Here's how the part is built. I have some questions about the finished solid (model axes, mm). Face numbers are marked on the shaded views. A direction names the side the tool comes from. Give positions to 0.01 mm unless a question says otherwise; leave off trailing zeros. Loops run counter-clockwise (first coordinate to the right, second up) from the corner with the lowest first, then second, coordinate; pieces in that order, holes last. Notation, with made-up numbers: M 73.5,55 L 77.5,55 A24 ccw 77.5,69 Z; hole C 73.5,31 d5. An arc over 180 degrees is marked long. Write item = value, one per line. Start each with the question number.
Autodesk Inventor part; units mm, degrees
ref_plane "YZ Plane" through (0, 0, 0) normal (1, 0, 0) x (0, 1, 0)
ref_plane "XZ Plane" through (0, 0, 0) normal (0, 1, 0) x (-1, 0, 0)
ref_plane "XY Plane" through (0, 0, 0) normal (0, 0, 1) x (1, 0, 0)
sketch "Sketch1" plane through (0, 0, 0) normal (0, 0, 1) x (1, 0, 0)
  line L0 (0, 0) -> (0, 25.4713) construction
  line L1 (-206.1253, 8.0706) -> (-206.1253, -17.3294)
  line L2 (-206.1253, -17.3294) -> (-203.2, -23.287)
  line L3 (-203.2, -23.287) -> (-203.2, -17.3294)
  line L4 (-203.2, -17.3294) -> (-196.85, -17.3294)
  line L5 (-196.85, -17.3294) -> (-196.85, -18.6213)
  line L6 (-206.1253, 8.0706) -> (-202.8327, 15.2137)
  line L7 (-202.8327, 15.2137) -> (-202.8327, 8.0706)
  line L8 (-202.8327, 8.0706) -> (-196.8015, 8.0706)
  line L9 (-196.8015, 8.0706) -> (-196.8015, 9.3626)
  line L10 (-196.8015, 9.3626) -> (-177.369, 9.3626)
  line L11 (-196.85, -18.6213) -> (-177.4174, -18.6213)
  line L12 (-159.6027, 47.4626) -> (-196.85, 47.4626)
  line L13 (-196.85, 47.4626) -> (-196.85, 71.7094)
  line L14 (-196.85, 71.7094) -> (-148.2962, 71.7094)
  line L15 (-159.6511, -56.7213) -> (-195.9938, -56.7213)
  line L16 (-195.9938, -56.7213) -> (-195.9938, -78.0553)
  line L17 (-195.9938, -78.0553) -> (-149.7029, -78.0553)
  line L18 (-177.369, 9.3626) -> (-159.6027, 47.4626)
  line L19 (-148.2962, 71.7094) -> (-143.6137, 81.751)
  line L20 (-177.4174, -18.6213) -> (-159.6511, -56.7213)
  line L21 (-149.7029, -78.0553) -> (-143.013, -92.4018)
  line L22 (-143.6137, 81.751) -> (-114.6581, 143.8464)
  line L23 (-143.013, -92.4018) -> (-109.7002, -163.8414)
  line L24 (-114.6581, 143.8464) -> (-88.6327, 143.8464)
  line L25 (-88.6327, 143.8464) -> (-88.6327, -163.8414)
  line L26 (-88.6327, -163.8414) -> (-109.7002, -163.8414)
  dimension "d0" = 6.35
  dimension "d3" = 203.2
  dimension "d11" = 38.1
  dimension "d12" = 38.1
  dimension "d13" = 0
  dimension "d14" = 25.4
  dimension "d15" = 0
  dimension "d16" = 115
  dimension "d17" = 115
revolve "Revolution1" add sketch "Sketch1" angle 360 about axis through (0, 0, 0) along (0, 1, 0)
properties part number "Section Adaptor WIP"
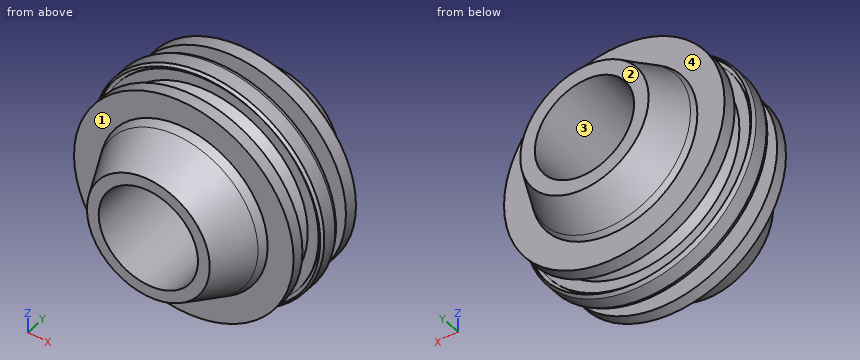
Q1. On a 3-axis mill with a long thin cutter (end or side, diameter ignored), from which of +Z, -Z, +X, -X, +Y, -Y can I reach the whole of each face in a straight line? I mean the marked faces 1 and 2. Say none if no direction works.
Q2. If we section it at A-A, the plane y = 55: List the corners of the cut face in (x, z) for me, then the cut area to 3 significant figures.
Q3. If we section it at B-B, the plane x = 164: State how many separate pieces and enclosed holes the cut face has, then the cut area to 3 significant figures.
Q4. If I drill on line 1 along Y through (x, z) = (140.5, -121); line 2 along Y through (x, z) = (50.5, 153); line 3 along Z through (x, y) = (0, 10.75), over which ranges is the centre line in solid material (lowest first)?
Q5. We'd pull the mould along Z, two halves only. Please class the marked faces 3 and 4: pulls with the +Z half, pulls with the -Z half, needs draft (parallel to the pull), parting line crosses it, or undercut.
Q6. If we section it at C-C, the plane y = 1: List the corners of the cut face in (x, z) for me.
Q7. Will these pins go through, and if not, where does the flat tip stop? pin 1 (12 mm diameter, centred on x = -49, y = 82, fed in from -Z); pin 2 (3 mm diameter, centred on x = -142.5, y = -55, fed in from +Z); pin 3 (3 mm diameter, centred on y = 51, z = -141.5, fed in from +X).
Resolved:
q1.face_1 = -Y
q1.face_2 = +Z, -Z, +X, -X, +Y
q2.outline = C 0,0 d393.7; hole C 0,0 d177.27
q2.area = 97,100 mm²
q3.separate_pieces = 3
q3.enclosed_holes = 0
q3.area = 22,000 mm²
q4.line_1 = -78.06 to -56.72, -18.62 to 9.36, 47.46 to 71.71
q4.line_2 = -78.06 to -56.72, -53.57 to 44.21, 47.46 to 71.71
q4.line_3 = -204.89 to -202.83, -176.72 to -88.63, 88.63 to 176.72, 202.83 to 204.89
q5.face_3 = undercut
q5.face_4 = needs draft
q6.outline = C 0,0 d412.25; hole C 0,0 d177.27
q7.pin_1 = -138.49
q7.pin_2 = 76.94
q7.pin_3 = 138.38
